Check sheet for the modelled part. Datum: model origin and axes. Units: mm. Give positions to 0.01 mm unless a question says otherwise; leave off trailing zeros. Write each loop counter-clockwise with the first axis right and the second up, starting at its lowest first coordinate (ties: lowest second). Pieces come first, ordered by that corner, then holes. Notation, with made-up numbers: (68.5, -19.5) -> (127.5, -19.5) arc R20 cw to (127.5, -7.5) -> close; hole circle Ø1 at (-20, 84.25). An arc over 180 degrees is marked (long way). Return JSON: item names as keys, results as strings.
from build123d import *

# Parameters (mm, degrees)
SKETCH1_W            = 88.9
SKETCH1_H            = 431.8
BOSS_EXTRUDE1_DEPTH  = 5.8
M3_CLEARANCE_HOLE1_D = 3.4
SKETCH2_W            = 38.1
SKETCH2_H            = 368.3
CUT_EXTRUDE1_DEPTH   = 441.89464728
SKETCH3_W            = 8.5
SKETCH3_H            = 431.8
BOSS_EXTRUDE2_DEPTH  = 5.8
SKETCH7_R            = 0.79375
CUT_EXTRUDE2_DEPTH   = 443.68684191
SKETCH9_W            = 25.4
SKETCH9_H            = 95.25
BOSS_EXTRUDE3_DEPTH  = 5.8
CUT_EXTRUDE3_DEPTH   = 449.959597291
SKETCH10_R           = 0.79375
CUT_EXTRUDE4_DEPTH   = 449.959597291
CUT_EXTRUDE5_DEPTH   = 449.959597291
FILLET1_R            = 5
FILLET2_R            = 6.35
SKETCH12_R           = 1.7272
CUT_EXTRUDE6_DEPTH   = 449.959597291


with BuildPart() as part:
    # Sketch1 → Boss-Extrude1 (new body)
    with BuildSketch(Plane(origin=(0, 0, 0), x_dir=(1, 0, 0), z_dir=(0, 1, 0))):
        with Locations((-44.45, -215.9)):
            Rectangle(SKETCH1_W, SKETCH1_H)
    extrude(amount=BOSS_EXTRUDE1_DEPTH)

    # M3 Clearance Hole1 (through all)
    with Locations(Plane(origin=(0, 5.8, 0), x_dir=(-1, 0, 0), z_dir=(0, 1, 0))):
        with Locations((82.55, 12.7), (6.35, 12.7), (6.35, 419.1), (82.55, 419.1), (82.55, 215.9), (6.35, 215.9)):
            Hole(M3_CLEARANCE_HOLE1_D / 2)

    # Sketch2 → Cut-Extrude1 (cut, through all)
    with BuildSketch(Plane(origin=(0, 5.8, 0), x_dir=(1, 0, 0), z_dir=(0, 1, 0))):
        with Locations((-44.45, -209.55)):
            Rectangle(SKETCH2_W, SKETCH2_H)
    extrude(amount=-CUT_EXTRUDE1_DEPTH, mode=Mode.SUBTRACT)

    # Sketch3 → Boss-Extrude2 (add, through all)
    with BuildSketch(Plane(origin=(0, 5.8, 0), x_dir=(-1, 0, 0), z_dir=(0, 1, 0))):
        with Locations((93.15, 215.9)):
            Rectangle(SKETCH3_W, SKETCH3_H)
    extrude(amount=-BOSS_EXTRUDE2_DEPTH)

    # Sketch7 → Cut-Extrude2 (cut, through all)
    with BuildSketch(Plane(origin=(0, 5.8, 0), x_dir=(1, 0, 0), z_dir=(0, 1, 0))):
        with Locations(Location((-44.45, -12.7, 0), (0, 0, 270))):
            Circle(SKETCH7_R)
        with Locations(Location((-82.55, -38.1, 0), (0, 0, 270))):
            Circle(SKETCH7_R)
        with Locations(Location((-6.35, -38.1, 0), (0, 0, 270))):
            Circle(SKETCH7_R)
        with Locations(Location((-6.35, -393.7, 0), (0, 0, 90))):
            Circle(SKETCH7_R)
        with Locations(Location((-82.55, -393.7, 0), (0, 0, 90))):
            Circle(SKETCH7_R)
        with Locations(Location((-44.45, -419.1, 0), (0, 0, 90))):
            Circle(SKETCH7_R)
    extrude(amount=-CUT_EXTRUDE2_DEPTH, mode=Mode.SUBTRACT)

    # Sketch9 → Boss-Extrude3 (add, through all)
    with BuildSketch(Plane(origin=(0, 5.8, 0), x_dir=(1, 0, 0), z_dir=(0, 1, 0))):
        with Locations((-110.1, -47.625)):
            Rectangle(SKETCH9_W, SKETCH9_H)
    extrude(amount=-BOSS_EXTRUDE3_DEPTH)

    # Sketch8 → Cut-Extrude3 (cut, through all)
    with BuildSketch(Plane(origin=(0, 5.8, 0), x_dir=(1, 0, 0), z_dir=(0, 1, 0))):
        with BuildLine():
            Line((-110.1, -44.45), (-113.275, -44.45))
            Line((-113.275, -44.45), (-113.275, -50.8))
            Line((-113.275, -50.8), (-110.1, -50.8))
            Line((-110.1, -50.8), (-110.1, -95.25))
            Line((-110.1, -95.25), (-97.4, -95.25))
            Line((-97.4, -95.25), (-97.4, -120.65))
            ThreePointArc((-97.4, -120.65), (-96.600813101, -110.993614483), (-94.225, -101.6))
            ThreePointArc((-94.225, -101.6), (-91.849186899, -92.206385517), (-91.05, -82.55))
            Line((-91.05, -82.55), (-91.05, -57.15))
            Line((-91.05, -57.15), (-100.575, -57.15))
            Line((-100.575, -57.15), (-100.575, -50.8))
            Line((-100.575, -50.8), (-97.4, -50.8))
            Line((-97.4, -50.8), (-97.4, -44.45))
            Line((-97.4, -44.45), (-100.575, -44.45))
            Line((-100.575, -44.45), (-100.575, -12.7))
            Line((-100.575, -12.7), (-110.1, -12.7))
            Line((-110.1, -12.7), (-110.1, -44.45))
        make_face()
    extrude(amount=-CUT_EXTRUDE3_DEPTH, mode=Mode.SUBTRACT)

    # Sketch10 → Cut-Extrude4 (cut, through all)
    with BuildSketch(Plane(origin=(0, 5.8, 0), x_dir=(1, 0, 0), z_dir=(0, 1, 0))):
        with Locations(Location((-116.45, -88.9, 0), (0, 0, 270))):
            Circle(SKETCH10_R)
        with Locations(Location((-116.45, -6.35, 0), (0, 0, 270))):
            Circle(SKETCH10_R)
    extrude(amount=-CUT_EXTRUDE4_DEPTH, mode=Mode.SUBTRACT)

    # Sketch11 → Cut-Extrude5 (cut, through all)
    with BuildSketch(Plane(origin=(0, 5.8, 0), x_dir=(1, 0, 0), z_dir=(0, 1, 0))):
        Polygon((-97.4, -414.3375), (-78.35, -414.3375), (-78.35, -420.6875), (-65.65, -420.6875), (-65.65, -404.8125), (-78.35, -404.8125), (-78.35, -411.1625), (-97.4, -411.1625), align=None)
    extrude(amount=-CUT_EXTRUDE5_DEPTH, mode=Mode.SUBTRACT)

    # Fillet1
    fillet1_edges = [part.edges().sort_by_distance(p)[0] for p in [
        (-97.4, 2.9, 411.1625),
    ]]
    fillet(fillet1_edges, radius=FILLET1_R)

    # Fillet2
    fillet2_edges = [part.edges().sort_by_distance(p)[0] for p in [
        (0, 2.9, 431.8),
        (-97.4, 2.9, 414.3375),
        (-97.4, 2.9, 431.8),
        (-122.8, 2.9, 95.25),
        (0, 2.9, 0),
        (-122.8, 2.9, 0),
        (-110.1, 2.9, 95.25),
    ]]
    fillet(fillet2_edges, radius=FILLET2_R - 0.0001)  # a hair under: the kernel refuses the full size

    # Sketch12 → Cut-Extrude6 (cut, through all)
    with BuildSketch(Plane.XZ):
        with Locations(Location((-69.45, 380.9, 0), (0, 0, 270))):
            Circle(SKETCH12_R)
        with Locations(Location((-19.45, 380.9, 0), (0, 0, 90))):
            Circle(SKETCH12_R)
        with Locations(Location((-69.45, 45.9, 0), (0, 0, 270))):
            Circle(SKETCH12_R)
        with Locations(Location((-19.45, 45.9, 0), (0, 0, 90))):
            Circle(SKETCH12_R)
    extrude(amount=-CUT_EXTRUDE6_DEPTH, mode=Mode.SUBTRACT)


solid = part.part
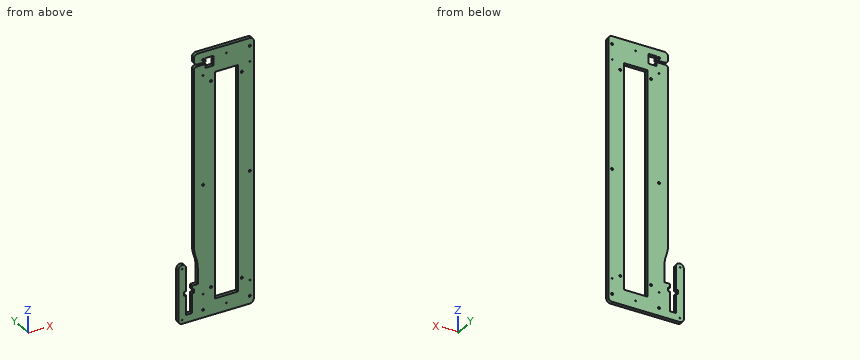
(1) Cross-section at C-C on y = 3.7. State how many separate pieces and enclosed holes the cut face has, then the cut area to 3 significant figures.
Reply:
{"separate pieces": "1", "enclosed holes": "19", "area": "28,800 mm^2"}
(2) Thickness scan on L1, parallel to X at y = 1.55, z = 38.1 (3 decimals); L2, parallel to X at y = 2.55, z = 45.9 (3 decimals); L3, parallel to Z at x = -26.5, y = 2.8. Record the ranges inside material, lowest first.
Reply:
{"L1": "-122.8 to -110.1, -100.575 to -83.344, -81.756 to -63.5, -25.4 to -7.144, -5.556 to 0", "L2": "-122.8 to -113.275, -97.4 to -71.177, -67.723 to -63.5, -25.4 to -21.177, -17.723 to 0", "L3": "0 to 25.4, 393.7 to 431.8"}
(3) Cross-section at B-B on x = -38.5. Enter the section's corners in (y, z).
Reply:
{"outline": "(0, 0) -> (5.8, 0) -> (5.8, 25.4) -> (0, 25.4) -> close; (0, 393.7) -> (5.8, 393.7) -> (5.8, 431.8) -> (0, 431.8) -> close"}
(4) Cross-section at A-A on z = 31. Enter the section's corners in (x, y) (3 decimals), then the cut area to 3 significant figures.
Reply:
{"outline": "(-122.8, 0) -> (-110.1, 0) -> (-110.1, 5.8) -> (-122.8, 5.8) -> close; (-100.575, 0) -> (-63.5, 0) -> (-63.5, 5.8) -> (-100.575, 5.8) -> close; (-25.4, 0) -> (0, 0) -> (0, 5.8) -> (-25.4, 5.8) -> close", "area": "436 mm^2"}
(5) Cross-section at D-D on x = -105.5. Enter the section's corners in (y, z), then the cut area to 3 significant figures.
Reply:
{"outline": "(0, 0) -> (5.8, 0) -> (5.8, 12.7) -> (0, 12.7) -> close", "area": "73.7 mm^2"}
